from build123d import *

# Parameters (mm, degrees)
EXTRUDE_THIN1_DEPTH = 2.54
EXTRUDE_THIN2_DEPTH = 6.35
BOSS_EXTRUDE1_DEPTH = 6.35
SKETCH2_R           = 31.75
BOSS_EXTRUDE2_DEPTH = 6.35
CUT_EXTRUDE1_DEPTH  = 6.35
SKETCH4_R           = 1
CUT_EXTRUDE2_DEPTH  = 16.24
CHAMFER2_SIZE       = 2.54


with BuildPart() as part:
    # Sketch1 → Extrude-Thin1 (new body)
    with BuildSketch(Plane.XY):
        with BuildLine():
            Line((-17.033098657, 5.209024178), (-9.398237952, 7.030294761))
            Line((-9.398237952, 7.030294761), (-6.628258472, 6.90375806))
            ThreePointArc((-6.628258472, 6.90375806), (-6.331733624, 7.041258836), (-6.201391634, 7.340999415))
            Line((-6.201391634, 7.340999415), (-6.07380581, 10.055084177))
            Line((-6.07380581, 10.055084177), (-3.543785692, 17.487046073))
            ThreePointArc((-3.543785692, 17.487046073), (0.967191009, 20.558965329), (5.170097171, 17.077417038))
            Line((5.170097171, 17.077417038), (6.991367754, 9.442556334))
            Line((6.991367754, 9.442556334), (6.864831053, 6.672576854))
            ThreePointArc((6.864831053, 6.672576854), (7.002331829, 6.376052005), (7.302072408, 6.245710016))
            Line((7.302072408, 6.245710016), (10.01615717, 6.118124192))
            Line((10.01615717, 6.118124192), (17.448119066, 3.588104073))
            ThreePointArc((17.448119066, 3.588104073), (20.520038322, -0.922872627), (17.038490031, -5.125778789))
            Line((17.038490031, -5.125778789), (9.401960539, -6.947447456))
            Line((9.401960539, -6.947447456), (6.687875777, -6.819861633))
            ThreePointArc((6.687875777, -6.819861633), (6.356638909, -6.939170255), (6.206783009, -7.257754026))
            Line((6.206783009, -7.257754026), (6.079197185, -9.971838788))
            Line((6.079197185, -9.971838788), (3.549177067, -17.403800684))
            ThreePointArc((3.549177067, -17.403800684), (-0.961799634, -20.47571994), (-5.164705796, -16.99417165))
            Line((-5.164705796, -16.99417165), (-6.986374463, -9.357642157))
            Line((-6.986374463, -9.357642157), (-6.85878864, -6.643557395))
            ThreePointArc((-6.85878864, -6.643557395), (-6.978097262, -6.312320527), (-7.296681033, -6.162464627))
            Line((-7.296681033, -6.162464627), (-10.010765795, -6.034878804))
            Line((-10.010765795, -6.034878804), (-17.442727691, -3.504858685))
            ThreePointArc((-17.442727691, -3.504858685), (-20.514646947, 1.006118016), (-17.033098657, 5.209024178))
        make_face()
        with BuildLine():
            Line((-16.443727069, 2.738347928), (-9.156812059, 4.476617225))
            Line((-9.156812059, 4.476617225), (-6.660884215, 4.362599602))
            ThreePointArc((-6.660884215, 4.362599602), (-4.589968036, 5.192045254), (-3.66419347, 7.221728815))
            Line((-3.66419347, 7.221728815), (-3.553485102, 9.576785873))
            Line((-3.553485102, 9.576785873), (-1.139293996, 16.66849877))
            ThreePointArc((-1.139293996, 16.66849877), (0.847920409, 18.021767165), (2.699420921, 16.488045451))
            Line((2.699420921, 16.488045451), (4.437690218, 9.201130441))
            Line((4.437690218, 9.201130441), (4.323672595, 6.705202597))
            ThreePointArc((4.323672595, 6.705202597), (5.153118247, 4.634286418), (7.182801808, 3.708511852))
            Line((7.182801808, 3.708511852), (9.537858866, 3.597803484))
            Line((9.537858866, 3.597803484), (16.629571763, 1.183612378))
            ThreePointArc((16.629571763, 1.183612378), (17.982840158, -0.803602027), (16.449118444, -2.655102539))
            Line((16.449118444, -2.655102539), (9.162203434, -4.393371836))
            Line((9.162203434, -4.393371836), (6.807146377, -4.282663469))
            ThreePointArc((6.807146377, -4.282663469), (4.646905931, -5.060763178), (3.669584845, -7.138483427))
            Line((3.669584845, -7.138483427), (3.558876477, -9.493540484))
            Line((3.558876477, -9.493540484), (1.144685371, -16.585253381))
            ThreePointArc((1.144685371, -16.585253381), (-0.842529034, -17.938521776), (-2.694029546, -16.404800062))
            Line((-2.694029546, -16.404800062), (-4.432298843, -9.117885052))
            Line((-4.432298843, -9.117885052), (-4.321590476, -6.762827995))
            ThreePointArc((-4.321590476, -6.762827995), (-5.099690185, -4.60258755), (-7.177410434, -3.625266463))
            Line((-7.177410434, -3.625266463), (-9.532467491, -3.514558095))
            Line((-9.532467491, -3.514558095), (-16.624180388, -1.100366989))
            ThreePointArc((-16.624180388, -1.100366989), (-17.977448783, 0.886847416), (-16.443727069, 2.738347928))
        make_face(mode=Mode.SUBTRACT)
    extrude(amount=EXTRUDE_THIN1_DEPTH)

    # Sketch1<5> → Extrude-Thin2 (add)
    with BuildSketch(Plane.XY):
        with BuildLine():
            Line((-17.033098657, 5.209024178), (-9.398237952, 7.030294761))
            Line((-9.398237952, 7.030294761), (-6.628258472, 6.90375806))
            ThreePointArc((-6.628258472, 6.90375806), (-6.331733624, 7.041258836), (-6.201391634, 7.340999415))
            Line((-6.201391634, 7.340999415), (-6.07380581, 10.055084177))
            Line((-6.07380581, 10.055084177), (-3.543785692, 17.487046073))
            ThreePointArc((-3.543785692, 17.487046073), (0.967191009, 20.558965329), (5.170097171, 17.077417038))
            Line((5.170097171, 17.077417038), (6.991367754, 9.442556334))
            Line((6.991367754, 9.442556334), (6.864831053, 6.672576854))
            ThreePointArc((6.864831053, 6.672576854), (7.002331829, 6.376052005), (7.302072408, 6.245710016))
            Line((7.302072408, 6.245710016), (10.01615717, 6.118124192))
            Line((10.01615717, 6.118124192), (17.448119066, 3.588104073))
            ThreePointArc((17.448119066, 3.588104073), (20.520038322, -0.922872627), (17.038490031, -5.125778789))
            Line((17.038490031, -5.125778789), (9.401960539, -6.947447456))
            Line((9.401960539, -6.947447456), (6.687875777, -6.819861633))
            ThreePointArc((6.687875777, -6.819861633), (6.356638909, -6.939170255), (6.206783009, -7.257754026))
            Line((6.206783009, -7.257754026), (6.079197185, -9.971838788))
            Line((6.079197185, -9.971838788), (3.549177067, -17.403800684))
            ThreePointArc((3.549177067, -17.403800684), (-0.961799634, -20.47571994), (-5.164705796, -16.99417165))
            Line((-5.164705796, -16.99417165), (-6.986374463, -9.357642157))
            Line((-6.986374463, -9.357642157), (-6.85878864, -6.643557395))
            ThreePointArc((-6.85878864, -6.643557395), (-6.978097262, -6.312320527), (-7.296681033, -6.162464627))
            Line((-7.296681033, -6.162464627), (-10.010765795, -6.034878804))
            Line((-10.010765795, -6.034878804), (-17.442727691, -3.504858685))
            ThreePointArc((-17.442727691, -3.504858685), (-20.514646947, 1.006118016), (-17.033098657, 5.209024178))
        make_face()
        with BuildLine():
            Line((-16.443727069, 2.738347928), (-9.156812059, 4.476617225))
            Line((-9.156812059, 4.476617225), (-6.660884215, 4.362599602))
            ThreePointArc((-6.660884215, 4.362599602), (-4.589968036, 5.192045254), (-3.66419347, 7.221728815))
            Line((-3.66419347, 7.221728815), (-3.553485102, 9.576785873))
            Line((-3.553485102, 9.576785873), (-1.139293996, 16.66849877))
            ThreePointArc((-1.139293996, 16.66849877), (0.847920409, 18.021767165), (2.699420921, 16.488045451))
            Line((2.699420921, 16.488045451), (4.437690218, 9.201130441))
            Line((4.437690218, 9.201130441), (4.323672595, 6.705202597))
            ThreePointArc((4.323672595, 6.705202597), (5.153118247, 4.634286418), (7.182801808, 3.708511852))
            Line((7.182801808, 3.708511852), (9.537858866, 3.597803484))
            Line((9.537858866, 3.597803484), (16.629571763, 1.183612378))
            ThreePointArc((16.629571763, 1.183612378), (17.982840158, -0.803602027), (16.449118444, -2.655102539))
            Line((16.449118444, -2.655102539), (9.162203434, -4.393371836))
            Line((9.162203434, -4.393371836), (6.807146377, -4.282663469))
            ThreePointArc((6.807146377, -4.282663469), (4.646905931, -5.060763178), (3.669584845, -7.138483427))
            Line((3.669584845, -7.138483427), (3.558876477, -9.493540484))
            Line((3.558876477, -9.493540484), (1.144685371, -16.585253381))
            ThreePointArc((1.144685371, -16.585253381), (-0.842529034, -17.938521776), (-2.694029546, -16.404800062))
            Line((-2.694029546, -16.404800062), (-4.432298843, -9.117885052))
            Line((-4.432298843, -9.117885052), (-4.321590476, -6.762827995))
            ThreePointArc((-4.321590476, -6.762827995), (-5.099690185, -4.60258755), (-7.177410434, -3.625266463))
            Line((-7.177410434, -3.625266463), (-9.532467491, -3.514558095))
            Line((-9.532467491, -3.514558095), (-16.624180388, -1.100366989))
            ThreePointArc((-16.624180388, -1.100366989), (-17.977448783, 0.886847416), (-16.443727069, 2.738347928))
        make_face(mode=Mode.SUBTRACT)
    extrude(amount=-EXTRUDE_THIN2_DEPTH)

    # Sketch1<6> → Boss-Extrude1 (add)
    with BuildSketch(Plane.XY):
        with BuildLine():
            ThreePointArc((-16.624180388, -1.100366989), (-17.977448783, 0.886847416), (-16.443727069, 2.738347928))
            Line((-16.443727069, 2.738347928), (-9.156812059, 4.476617225))
            Line((-9.156812059, 4.476617225), (-6.660884215, 4.362599602))
            ThreePointArc((-6.660884215, 4.362599602), (-4.589968036, 5.192045254), (-3.66419347, 7.221728815))
            Line((-3.66419347, 7.221728815), (-3.553485102, 9.576785873))
            Line((-3.553485102, 9.576785873), (-1.139293996, 16.66849877))
            ThreePointArc((-1.139293996, 16.66849877), (0.847920409, 18.021767165), (2.699420921, 16.488045451))
            Line((2.699420921, 16.488045451), (4.437690218, 9.201130441))
            Line((4.437690218, 9.201130441), (4.323672595, 6.705202597))
            ThreePointArc((4.323672595, 6.705202597), (5.153118247, 4.634286418), (7.182801808, 3.708511852))
            Line((7.182801808, 3.708511852), (9.537858866, 3.597803484))
            Line((9.537858866, 3.597803484), (16.629571763, 1.183612378))
            ThreePointArc((16.629571763, 1.183612378), (17.982840158, -0.803602027), (16.449118444, -2.655102539))
            Line((16.449118444, -2.655102539), (9.162203434, -4.393371836))
            Line((9.162203434, -4.393371836), (6.807146377, -4.282663469))
            ThreePointArc((6.807146377, -4.282663469), (4.646905931, -5.060763178), (3.669584845, -7.138483427))
            Line((3.669584845, -7.138483427), (3.558876477, -9.493540484))
            Line((3.558876477, -9.493540484), (1.144685371, -16.585253381))
            ThreePointArc((1.144685371, -16.585253381), (-0.842529034, -17.938521776), (-2.694029546, -16.404800062))
            Line((-2.694029546, -16.404800062), (-4.432298843, -9.117885052))
            Line((-4.432298843, -9.117885052), (-4.321590476, -6.762827995))
            ThreePointArc((-4.321590476, -6.762827995), (-5.099690185, -4.60258755), (-7.177410434, -3.625266463))
            Line((-7.177410434, -3.625266463), (-9.532467491, -3.514558095))
            Line((-9.532467491, -3.514558095), (-16.624180388, -1.100366989))
        make_face()
    extrude(amount=-BOSS_EXTRUDE1_DEPTH)

    # Sketch2 → Boss-Extrude2 (add)
    with BuildSketch(Plane(origin=(0, 0, -6.35), x_dir=(-1, 0, 0), z_dir=(0, 0, -1))):
        Circle(SKETCH2_R)
    extrude(amount=BOSS_EXTRUDE2_DEPTH)

    # Sketch3 → Cut-Extrude1 (cut)
    with BuildSketch(Plane(origin=(0, 0, -12.7), x_dir=(-1, 0, 0), z_dir=(0, 0, -1))):
        with BuildLine():
            Line((-16.934288716, 16.934288716), (-12.444160656, 12.444160656))
            ThreePointArc((-12.444160656, 12.444160656), (0, 17.598700771), (12.444160656, 12.444160656))
            Line((12.444160656, 12.444160656), (16.934288716, 16.934288716))
            ThreePointArc((16.934288716, 16.934288716), (0, 23.948700771), (-16.934288716, 16.934288716))
        make_face()
        with BuildLine():
            Line((6.198379865, -23.132668581), (4.554878929, -16.999039584))
            ThreePointArc((4.554878929, -16.999039584), (15.240921942, -8.799350386), (16.999039584, 4.554878929))
            Line((16.999039584, 4.554878929), (23.132668581, 6.198379865))
            ThreePointArc((23.132668581, 6.198379865), (20.740183256, -11.974350386), (6.198379865, -23.132668581))
        make_face()
        with BuildLine():
            Line((-23.132668581, 6.198379865), (-16.999039584, 4.554878929))
            ThreePointArc((-16.999039584, 4.554878929), (-15.240921942, -8.799350386), (-4.554878929, -16.999039584))
            Line((-4.554878929, -16.999039584), (-6.198379865, -23.132668581))
            ThreePointArc((-6.198379865, -23.132668581), (-20.740183256, -11.974350386), (-23.132668581, 6.198379865))
        make_face()
    extrude(amount=-CUT_EXTRUDE1_DEPTH, mode=Mode.SUBTRACT)

    # Sketch4 → Cut-Extrude2 (cut, through all)
    with BuildSketch(Plane(origin=(0, 0, -12.7), x_dir=(-1, 0, 0), z_dir=(0, 0, -1))):
        Circle(SKETCH4_R)
    extrude(amount=-CUT_EXTRUDE2_DEPTH, mode=Mode.SUBTRACT)

    # Chamfer2
    chamfer2_edges = [part.edges().sort_by_distance(p)[0] for p in [
        (1, 0, -12.7),
    ]]
    chamfer(chamfer2_edges, length=CHAMFER2_SIZE)


solid = part.part
Source: CAD feature listing. Evaluate the final solid. Frame: model axes, mm. A direction names the side the tool comes from. Coordinates: 2 decimals unless noted, no trailing zeros. Loops run counter-clockwise (first coordinate to the right, second up) from the corner with the lowest first, then second, coordinate; pieces in that order, holes last. Notation, with made-up numbers: (-32.5, 88.5) - (20.5, 88.5) arc R35 ccw to (20.5, 121.5) - close; hole circle Ø6 at (-39.5, 29). An arc over 180 degrees is marked (long way). Return JSON: item names as keys, results as strings.
Q1. Material intervals for line 1 along Y through (x, z) = (0, -7.25); line 2 along X through (y, z) = (-3.5, -10.25); line 3 along Z through (x, y) = (-19, 9), sorted ascending.
Results:
{"line 1": "-31.75 to -1, 1 to 17.6, 23.95 to 31.75", "line 2": "-31.56 to -23.69, -17.25 to 17.25, 23.69 to 31.56", "line 3": "-12.7 to -6.35"}
Q2. Section D-D, the plane z = -11.25. Return loops of the section in (x, y).
Results:
{"outline": "circle Ø63.5 at (0, 0); hole (-23.13, 6.2) arc R23.95 ccw to (-6.2, -23.13) - (-4.55, -17) arc R17.6 cw to (-17, 4.55) - close; hole (-16.93, 16.93) - (-12.44, 12.44) arc R17.6 cw to (12.44, 12.44) - (16.93, 16.93) arc R23.95 ccw to start; hole circle Ø4.18 at (0, 0); hole (4.55, -17) - (6.2, -23.13) arc R23.95 ccw to (23.13, 6.2) - (17, 4.55) arc R17.6 cw to start"}
Q3. Section B-B, the plane z = -1.25. Return loops of the section in (x, y), plus the area to 3 significant figures.
Results:
{"outline": "(-17.44, -3.5) - (-10.01, -6.03) - (-7.3, -6.16) arc R0.46 cw to (-6.86, -6.64) - (-6.99, -9.36) - (-5.16, -16.99) arc R4.54 ccw to (3.55, -17.4) - (6.08, -9.97) - (6.21, -7.26) arc R0.46 cw to (6.69, -6.82) - (9.4, -6.95) - (17.04, -5.13) arc R4.54 ccw to (17.45, 3.59) - (10.02, 6.12) - (7.3, 6.25) arc R0.46 cw to (6.86, 6.67) - (6.99, 9.44) - (5.17, 17.08) arc R4.54 ccw to (-3.54, 17.49) - (-6.07, 10.06) - (-6.2, 7.34) arc R0.46 cw to (-6.63, 6.9) - (-9.4, 7.03) - (-17.03, 5.21) arc R4.54 ccw to start; hole circle Ø2 at (0, 0)", "area": "748 mm2"}
Q4. Mould query, pull axis Y, two halves, no side actions, for faces 6 (the flat face through (-13.3, 6.1, -1.8)), 7 (the cylindrical face through (17.984, -0.768, 1.288)), 8 (the flat face through (-8.6, -6.1, -1.8)). Classes: released by +Y, released by -Y, zero draft, split by the parting line, or undercut.
Results:
{"face 6": "released by +Y", "face 7": "undercut", "face 8": "released by -Y"}
Q5. Section A-A, the plane y = 0. Return loops of the section in (x, z), plus the area to 3 significant figures.
Results:
{"outline": "(-31.75, -12.7) - (-23.95, -12.7) - (-23.95, -6.35) - (-31.75, -6.35) - close; (-20.45, -6.35) - (-17.6, -6.35) - (-17.6, -12.7) - (-3.54, -12.7) - (-1, -10.16) - (-1, 0) - (-17.82, 0) - (-17.82, 2.54) - (-20.45, 2.54) - close; (1, -10.16) - (3.54, -12.7) - (17.6, -12.7) - (17.6, -6.35) - (20.47, -6.35) - (20.47, 2.54) - (17.85, 2.54) - (17.85, 0) - (1, 0) - close; (23.95, -12.7) - (31.75, -12.7) - (31.75, -6.35) - (23.95, -6.35) - close", "area": "564 mm2"}
Q6. Section C-C, the plane y = -21.5. Return loops of the section in (x, z).
Results:
{"outline": "(-23.36, -12.7) - (-10.55, -12.7) - (-10.55, -6.35) - (-23.36, -6.35) - close; (-5.76, -12.7) - (5.76, -12.7) - (5.76, -6.35) - (-5.76, -6.35) - close; (10.55, -12.7) - (23.36, -12.7) - (23.36, -6.35) - (10.55, -6.35) - close"}
Q7. Access query for faces 1 (the flat face through (20.11, 5.39, -9.57)), 2 (the flat face through (-20.023, 5.365, -9.569)), 3 (the flat face through (-8.033, 6.968, -1.843)), 4 (the flat face through (-3.61, 8.38, 1.29)), 5 (the flat face through (6.93, 8.08, -1.84)). Directions: +Z, -Z, +X, -X, +Y, -Y. A direction counts if a zero-diameter tool reaches every point of the face in a straight line with its end or side. Return the directions, or none.
Results:
{"face 1": "+Z, -Z", "face 2": "-Z", "face 3": "+Z, +Y", "face 4": "+Z", "face 5": "+Z, +X"}
Q8. Contact query for flat-ended pins moving along their axis: P1, Ø5, axis at x = 19.5, z = -1, coming from the -Y side; P2, Ø4, axis at y = -16, z = 0.5, coming from the +X side; P3, Ø1.1, axis at x = -19.5, y = 1.5, coming from the -Z side. Output: stop coordinate, or through.
Results:
{"P1": "y = -5.13", "P2": "x = 4.71", "P3": "z = -6.35"}
